The listing builds one solid part. Answer for the finished solid, in the listing's coordinates (mm). Face numbers are marked on the shaded views. A direction names the side the tool comes from. Give positions to 0.01 mm unless a question says otherwise; leave off trailing zeros. Write each loop counter-clockwise with the first axis right and the second up, starting at its lowest first coordinate (ties: lowest second). Pieces come first, ordered by that corner, then holes. Notation, with made-up numbers: (-14, 56) -> (18, 56) arc R14 cw to (18, 61) -> close; hole circle Ø3 at (81.25, -31). An arc over 180 degrees is marked (long way). Put each result on its own line as item: value. Start each with the question number.
1) A cutting plane is placed at C-C (x = -44.5). Write down the section's boundary in (y, z).
2) For the marked faces 1, 2 and 3, determine the directions among +Z, -Z, +X, -X, +Y, -Y from which every point of the face is accessible in a straight line to the end or side of a thin tool.
3) A cutting plane is placed at A-A (y = -15). Write down the section's boundary in (x, z).
4) For a pull along Z with two mould halves and no side action, classify the marked faces 4, 5 and 6 as released by +Z, released by -Z, zero draft, split by the parting line, or undercut.
5) A cutting plane is placed at D-D (y = 2). Write down the section's boundary in (x, z), then the cut area to 3 significant figures.
6) A cutting plane is placed at B-B (z = -50). Write down the section's boundary in (x, y).
7) Flat-ended cylindrical pins translate along their axes: pin 1 Ø8 at (x, y) = (-31.5, 6.5) entering from +Z; pin 2 Ø10 at (y, z) = (0, -42) entering from +X; pin 3 Ø2 at (y, z) = (-21.5, -65.5) entering from +X. Find the tip coordinate at first contact, or state that the pin passes through.
8) Find the intervals of material crossed by line 1 along Z through (x, y) = (-82.25, -15); line 2 along Y through (x, z) = (-40, -43.5); line 3 along X through (y, z) = (10, -46), in increasing order. Write a range as from..to.
Autodesk Inventor part; units mm, degrees
ref_plane "YZ Plane" through (0, 0, 0) normal (1, 0, 0) x (0, 1, 0)
ref_plane "XZ Plane" through (0, 0, 0) normal (0, 1, 0) x (-1, 0, 0)
ref_plane "XY Plane" through (0, 0, 0) normal (0, 0, 1) x (1, 0, 0)
sketch "Sketch1" plane through (0, 0, 0) normal (0, 1, 0) x (-1, 0, 0)
  circle A0 centre (50.2019, -50) radius 25
  point P0 (0, 0)
  dimension "d0" = 50
  dimension "d1" = 50
extrude "Extrusion1" add sketch "Sketch1" along normal blind 20
sketch "Sketch2" plane through (-50.2019, 20, -50) normal (0, 1, 0) x (1, 0, 0)
  line L0 (-35, -15) -> (-16.3886, -15)
  line L1 (-16.3886, -15) -> (-16.3886, 15)
  line L2 (-16.3886, 15) -> (-35, 15)
  line L3 (-35, 15) -> (-35, -15)
  circle A0 centre (0, 0) radius 25
  circle A1 centre (0, 0) radius 25
  point P0 (50.2019, -50)
  point P1 (0, 25)
  point P2 (0, -25)
  point P3 (-20, -15)
  point P4 (-20, 15)
  dimension "d4" = 15
  dimension "d5" = 15
  dimension "d6" = 35
  dimension "d7" = 50
extrude "Extrusion2" add sketch "Sketch2" against normal blind 50 contours L3 L2 A0 L0
sketch "Sketch3" plane through (0, 0, 0) normal (0, -1, 0) x (1, 0, 0)
  arc A0 (-70.2019, -65) -> (-70.2019, -35) centre (-50.2019, -50) ccw
  arc A1 (-70.2019, -35) -> (-70.2019, -65) centre (-50.2019, -50) ccw
  circle A2 centre (-50.2019, -50) radius 7.5
  point P0 (0, 0)
  point P1 (-50.2019, -75)
  point P2 (-50.2019, -25)
  point P3 (-75.2019, -50)
  point P4 (-25.01, -50)
  dimension "d10" = 15
  dimension "d11" = 25
extrude "Extrusion3" cut sketch "Sketch3" against normal blind 30 contours A2
sketch "Sketch4" plane through (-85.2019, 20, -65) normal (-1, 0, 0) x (0, 0, 1)
  line L0 (0, -20) -> (0, -50)
  line L1 (30, -20) -> (30, -50)
  line L2 (30, -50) -> (0, -50)
  line L3 (40, -20) -> (-10, -20)
  circle A0 centre (15, -35) radius 6
  point P0 (65, -20)
  point P1 (0, -35)
  point P2 (30, -35)
  point P3 (15, -50)
  point P4 (15, -20)
  point P5 (15, -20)
  dimension "d14" = 30
  dimension "d15" = 15
  dimension "d16" = 15
  dimension "d17" = 12
extrude "Extrusion4" cut sketch "Sketch4" against normal blind 30 contours A0
equation "\"d10\" = 0.6 * d11"
equation "\"d17\" = 0.4 * d14"
properties part number "KeelHook"
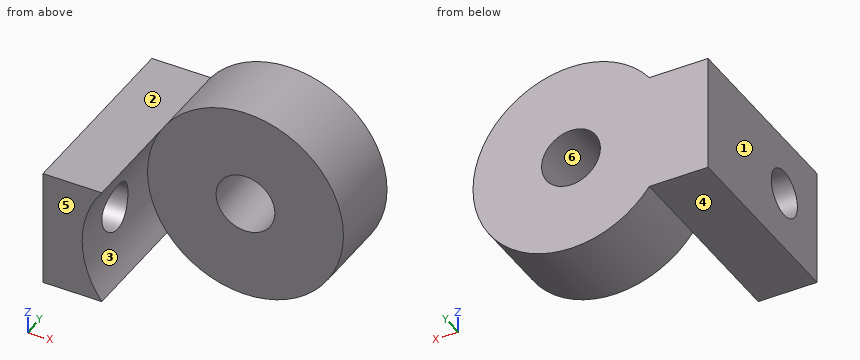
Reply:
1. outline: (0, -74.34) -> (20, -74.34) -> (20, -54.87) -> (0, -54.87) -> close; (0, -45.13) -> (20, -45.13) -> (20, -25.66) -> (0, -25.66) -> close
2. face 1: +Z, -Z, -X, +Y, -Y
2. face 2: +Z, -X, +Y, -Y
2. face 3: +X, -Y
3. outline: (-85.2, -65) -> (-70.2, -65) arc R25 cw to (-74.47, -56) -> (-85.2, -56) -> close; (-85.2, -44) -> (-74.47, -44) arc R25 cw to (-70.2, -35) -> (-85.2, -35) -> close
4. face 4: released by -Z
4. face 5: zero draft
4. face 6: undercut
5. outline: (-85.2, -65) -> (-70.2, -65) arc R25 ccw (long way) to (-70.2, -35) -> (-85.2, -35) -> close; hole circle Ø15 at (-50.2, -50)
5. area: 2,130 mm2
6. outline: (-85.2, -30) -> (-75.2, -30) -> (-75.2, -21) -> (-85.2, -21) -> close; (-85.2, -9) -> (-75.2, -9) -> (-75.2, 0) -> (-57.7, 0) -> (-57.7, 20) -> (-85.2, 20) -> close; (-42.7, 0) -> (-25.2, 0) -> (-25.2, 20) -> (-42.7, 20) -> close
7. pin 1: stops at z = -29.78
7. pin 2: stops at x = -25.38
7. pin 3: stops at x = -70.2
8. line 1: z = -65..-56, -44..-35
8. line 2: y = 0..20
8. line 3: x = -85.2..-56.55, -43.86..-25.52
